Drawing for the job (mm, zero at the part's lowest x, y, z). A direction names the side the tool comes from. Give positions to 0.01 mm unless a question says otherwise; leave off trailing zeros. Order: outer loops, then holes, each group sorted by start corner. A loop starts at its lowest first (then second) coordinate and runs counter-clockwise, first axis right, second up. Notation, with made-up numbers: M -26,85 L 3,85 A15 cw 3,97 Z; hole C 15.5,28 d9. An arc over 180 degrees is marked long. Answer as a JSON object with one key per item and string values.
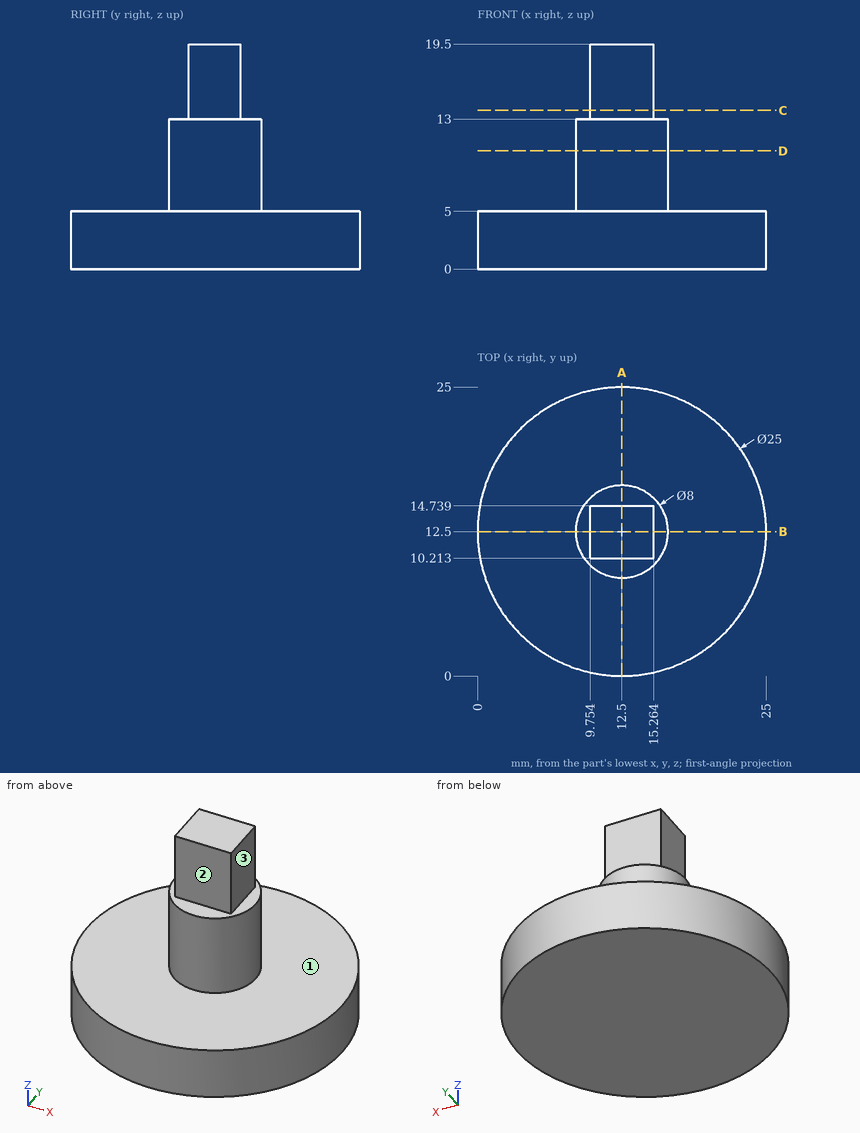
1. Cut at A-A on x = 12.5. Give the cut face in (y, z).
Worked answers:
{"outline": "M 0,0 L 25,0 L 25,5 L 16.5,5 L 16.5,13 L 14.74,13 L 14.74,19.5 L 10.21,19.5 L 10.21,13 L 8.5,13 L 8.5,5 L 0,5 Z"}
2. Cut at D-D on z = 10.25. Give the cut face in (x, y).
Worked answers:
{"outline": "C 12.5,12.5 d8"}
3. Which spindle directions (+Z, -Z, +X, -X, +Y, -Y) get a long thin tool onto all of the face, cutting with end or side? Do the marked faces 1, 2 and 3. Say none if no direction does.
Worked answers:
{"face 1": "+Z", "face 2": "+Z, +X, -X, -Y", "face 3": "+Z, +X, +Y, -Y"}
4. Cut at B-B on y = 12.5. Give the cut face in (x, z).
Worked answers:
{"outline": "M 0,0 L 25,0 L 25,5 L 16.5,5 L 16.5,13 L 15.26,13 L 15.26,19.5 L 9.75,19.5 L 9.75,13 L 8.5,13 L 8.5,5 L 0,5 Z"}
5. Pin check, flat tips, straight feed: P1, Ø2.5, axis at y = 11.5, z = 16, coming from the +X side; P2, Ø1.5, axis at y = 12, z = 6.5, coming from the -X side; P3, Ø10, axis at y = 5, z = 11.5, coming from the +X side. Stop position of each tip, or through.
Worked answers:
{"P1": "stops at x = 15.26", "P2": "stops at x = 8.5", "P3": "stops at x = 15.62"}
6. Probe line 1 along Z through (x, y) = (18.75, 6.5); line 2 along Z through (x, y) = (13.25, 16); line 3 along Y through (x, z) = (14, 15.5). List the from-to ranges inside material, lowest first.
Worked answers:
{"line 1": "z = 0 to 5", "line 2": "z = 0 to 13", "line 3": "y = 10.21 to 14.74"}
7. Cut at C-C on z = 13.75. Give the cut face in (x, y).
Worked answers:
{"outline": "M 9.75,10.21 L 15.26,10.21 L 15.26,14.74 L 9.75,14.74 Z"}
